Could you check a few things on this model? Use its own coordinates, in mm. Face numbers are marked on the shaded views. A direction names the side the tool comes from. Coordinates: 2 decimals unless noted, no trailing zeros. Order: outer loops, then holes, each group sorted by start corner. A loop starts at its lowest first (then second) coordinate and runs counter-clockwise, first axis right, second up. Notation, with made-up numbers: (46, 49.5) - (72, 49.5) arc R7 cw to (72, 61.5) - close; hole circle Ø8 at (44, -12). An arc over 180 degrees is marked (long way). Answer as CSV lines item,"result". Start each with the question number.
1. For the marked faces 4 and 5, which set-ups out of +Z, -Z, +X, -X, +Y, -Y let a thin tool reach every point of the face, with its end or its side?
2. Thinking about a two-plate mould opening in Z: for the marked faces 1, 2 and 3, which applies, released by +Z, released by -Z, zero draft, split by the parting line, or undercut?
3. I want a section at B-B, the plane z = 1. List the corners of the cut face in (x, y) for me, and give its area (3 significant figures).
4. I want a section at A-A, the plane y = 0.75. List the corners of the cut face in (x, z) for me, and give its area (3 significant figures).
5. For pin 1 (6.5 mm diameter, centred on x = 0.5, z = -0.5, fed in from +Y), with a flat end and sliding along its axis, tell me the tip position at first contact or that it passes through.
6. I need wall thicknesses on probe 1 along Y at (x, z) = (3.75, -0.5); probe 2 along Z at (x, y) = (-1, 1.6); probe 3 along X at (y, z) = (0.75, -3.25). Which ranges of each line are inside material? Lowest first, please.
7. I want a section at C-C, the plane x = -2. List the corners of the cut face in (y, z) for me, and give its area (3 significant figures).
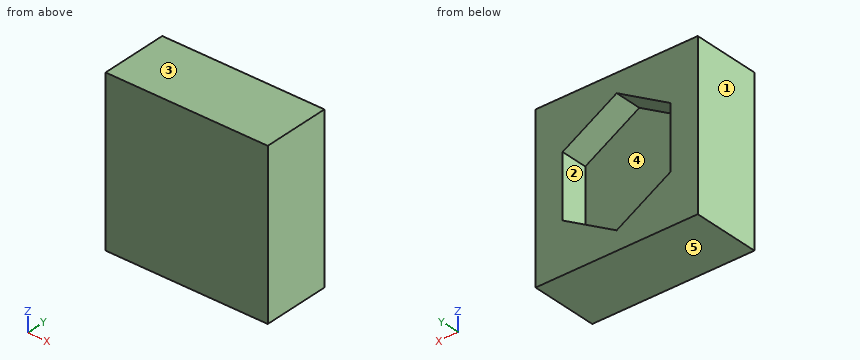
Autodesk Inventor part; units mm, degrees
ref_plane "YZ Plane" through (0, 0, 0) normal (1, 0, 0) x (0, 1, 0)
ref_plane "XZ Plane" through (0, 0, 0) normal (0, 1, 0) x (-1, 0, 0)
ref_plane "XY Plane" through (0, 0, 0) normal (0, 0, 1) x (1, 0, 0)
sketch "Sketch1" plane through (0, 0, 0) normal (0, 1, 0) x (-1, 0, 0)
  line L0 (-6, 6) -> (6, 6)
  line L1 (6, 6) -> (6, -6)
  line L2 (6, -6) -> (-6, -6)
  line L3 (-6, -6) -> (-6, 6)
  line L4 (-6, 6) -> (6, -6) construction
  line L5 (6, 6) -> (-6, -6) construction
  point P0 (0, 0)
  dimension "d0" = 12
  dimension "d1" = 12
extrude "Extrusion1" add sketch "Sketch1" along normal mid plane 5
sketch "Sketch2" plane through (0, 2.5, 0) normal (0, 1, 0) x (1, 0, 0)
  line L0 (-4, 2.3094) -> (0, 4.6188)
  line L1 (0, 4.6188) -> (4, 2.3094)
  line L2 (4, 2.3094) -> (4, -2.3094)
  line L3 (4, -2.3094) -> (0, -4.6188)
  line L4 (0, -4.6188) -> (-4, -2.3094)
  line L5 (-4, -2.3094) -> (-4, 2.3094)
  point P0 (0, 0)
  point P1 (0, 0)
  dimension "d8" = 8
extrude "Extrusion2" cut sketch "Sketch2" against normal blind 2
equation "\"d1\" = d0"
properties part number "PressFItTestHole"
Solved:
1,face 4,"+Y"
1,face 5,"-Z, +X, -X, +Y, -Y"
2,face 1,"zero draft"
2,face 2,"undercut"
2,face 3,"released by +Z"
3,outline,"(-6, -2.5) - (6, -2.5) - (6, 2.5) - (4, 2.5) - (4, 0.5) - (-4, 0.5) - (-4, 2.5) - (-6, 2.5) - close"
3,area,"44.0 mm2"
4,outline,"(-6, -6) - (6, -6) - (6, 6) - (-6, 6) - close; hole (-4, -2.31) - (0, -4.62) - (4, -2.31) - (4, 2.31) - (0, 4.62) - (-4, 2.31) - close"
4,area,"88.6 mm2"
5,pin 1,"stops at y = 0.5"
6,probe 1,"y = -2.5 to 0.5"
6,probe 2,"z = -6 to -4.04, 4.04 to 6"
6,probe 3,"x = -6 to -2.37, 2.37 to 6"
7,outline,"(-2.5, -6) - (2.5, -6) - (2.5, -3.46) - (0.5, -3.46) - (0.5, 3.46) - (2.5, 3.46) - (2.5, 6) - (-2.5, 6) - close"
7,area,"46.1 mm2"
